Part model, mm, in its own coordinate system. Face numbers are marked on the shaded views. A direction names the side the tool comes from. Round coordinates to 2 decimals unless told otherwise and drop trailing zeros. Loops run counter-clockwise (first coordinate to the right, second up) from the corner with the lowest first, then second, coordinate; pieces in that order, holes last. Notation, with made-up numbers: M 66,-4 L 119,-4 A12 cw 119,2 Z; hole C -26,-19.5 d4. An arc over 180 degrees is marked long. Put each result on its own line as item: value. Start each with the question number.
1) Probe line 1 along Y through (x, z) = (0, 1.4) (3 decimals); line 2 along X through (y, z) = (-2, 1.5); line 3 along Y through (x, z) = (10, 5) (3 decimals). List the from-to ranges inside material, lowest first.
2) Which spindle directions (+Z, -Z, +X, -X, +Y, -Y) get a long thin tool onto all of the face, cutting with end or side? Do the marked faces 1, 2 and 3. Say none if no direction does.
3) Slice it at A-A on y = 0. Give the cut face in (x, z) (3 decimals), then the cut area to 3 significant figures.
4) Pull direction X, two halves, no side cores. Call the marked faces 4, 5, 6 and 7: +X half, -X half, draft (parallel to the pull), parting line (faces both ways), or undercut.
5) Slice it at C-C on z = 4.75. Give the cut face in (x, y) (3 decimals), then the cut area to 3 significant figures.
6) Slice it at D-D on x = -18. Give the cut face in (y, z), then the cut area to 3 significant figures.
7) Drop flat-ended pins along their axis: pin 1 Ø5 at (x, y) = (-17.5, -17.5) entering from -Z; pin 2 Ø4 at (x, y) = (0, 10) entering from +Z; pin 3 Ø2.5 at (x, y) = (-12.73, 12.73) entering from +Z; pin 4 Ø1.8 at (x, y) = (0, -1.5) entering from -Z. Give the stop position or say it passes through.
```python
from build123d import *

# Parameters (mm, degrees)
ESQUISSE1_R             = 24
ESQUISSE1_R_2           = 1.5
ESQUISSE1_R_3           = 3
BOSS_EXTRU_1_DEPTH      = 4
ESQUISSE2_R             = 14.85
BOSS_EXTRU_2_DEPTH      = 7
ESQUISSE3_R             = 2.375
ENL_V_MAT_EXTRU_1_DEPTH = 10


with BuildPart() as part:
    # Esquisse1 → Boss.-Extru.1 (new body)
    with BuildSketch(Plane.XY):
        Circle(ESQUISSE1_R)
        with Locations((0, 18)):
            Circle(ESQUISSE1_R_2, mode=Mode.SUBTRACT)
        with Locations((12.727922061, 12.727922061)):
            Circle(ESQUISSE1_R_2, mode=Mode.SUBTRACT)
        with Locations((18, 0)):
            Circle(ESQUISSE1_R_2, mode=Mode.SUBTRACT)
        with Locations((12.727922061, -12.727922061)):
            Circle(ESQUISSE1_R_2, mode=Mode.SUBTRACT)
        with Locations((0, -18)):
            Circle(ESQUISSE1_R_2, mode=Mode.SUBTRACT)
        with Locations((-12.727922061, -12.727922061)):
            Circle(ESQUISSE1_R_2, mode=Mode.SUBTRACT)
        with Locations((-18, 0)):
            Circle(ESQUISSE1_R_2, mode=Mode.SUBTRACT)
        with Locations((-12.727922061, 12.727922061)):
            Circle(ESQUISSE1_R_2, mode=Mode.SUBTRACT)
        Circle(ESQUISSE1_R_3, mode=Mode.SUBTRACT)
    extrude(amount=BOSS_EXTRU_1_DEPTH)

    # Esquisse2 → Boss.-Extru.2 (add)
    with BuildSketch(Plane.XY.offset(4)):
        Circle(ESQUISSE2_R)
    extrude(amount=BOSS_EXTRU_2_DEPTH)

    # Esquisse3 → Enlèv. mat.-Extru.1 (cut)
    with BuildSketch(Plane.XY.offset(11)):
        with Locations((0, 10)):
            Circle(ESQUISSE3_R)
        with Locations((10, 0)):
            Circle(ESQUISSE3_R)
        with Locations((0, -10)):
            Circle(ESQUISSE3_R)
        with Locations((-10, 0)):
            Circle(ESQUISSE3_R)
    extrude(amount=-ENL_V_MAT_EXTRU_1_DEPTH, mode=Mode.SUBTRACT)


solid = part.part
```
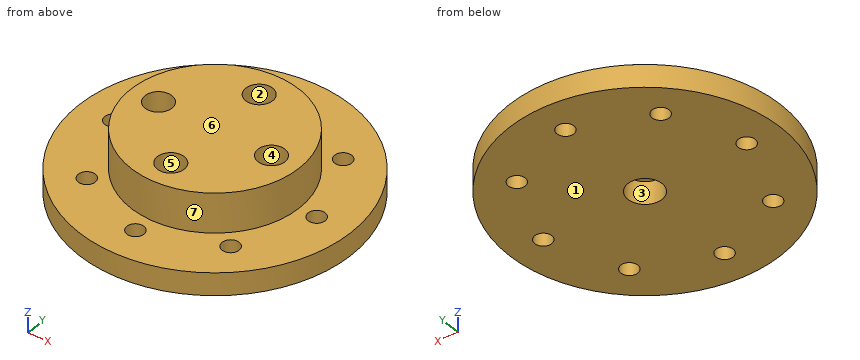
Recorded:
1. line 1: y = -24 to -19.5, -16.5 to -12.375, -7.625 to -3, 3 to 7.625, 12.375 to 16.5, 19.5 to 24
1. line 2: x = -23.92 to -11.28, -8.72 to -2.24, 2.24 to 8.72, 11.28 to 23.92
1. line 3: y = -10.978 to -2.375, 2.375 to 10.978
2. face 1: -Z, +X, -X, +Y, -Y
2. face 2: +Z
2. face 3: -Z
3. outline: M -24,0 L -19.5,0 L -19.5,4 L -24,4 Z; M -16.5,0 L -3,0 L -3,4 L 3,4 L 3,0 L 16.5,0 L 16.5,4 L 14.85,4 L 14.85,11 L 12.375,11 L 12.375,1 L 7.625,1 L 7.625,11 L -7.625,11 L -7.625,1 L -12.375,1 L -12.375,11 L -14.85,11 L -14.85,4 L -16.5,4 Z; M 19.5,0 L 24,0 L 24,4 L 19.5,4 Z
3. area: 257 mm2
4. face 4: undercut
4. face 5: undercut
4. face 6: draft
4. face 7: parting line
5. outline: C 0,0 d29.7; hole C -10,0 d4.75; hole C 0,-10 d4.75; hole C 0,10 d4.75; hole C 10,0 d4.75
5. area: 622 mm2
6. outline: M -15.87,0 L -1.5,0 L -1.5,4 L -15.87,4 Z; M 1.5,0 L 15.87,0 L 15.87,4 L 1.5,4 Z
6. area: 115 mm2
7. pin 1: stops at z = 0
7. pin 2: stops at z = 1
7. pin 3: passes through
7. pin 4: stops at z = 4
